Geometry check sheet. Reference: drawing and pictorial views, mm from the part's lowest x, y, z. A direction names the side the tool comes from. Give positions to 0.01 mm unless a question says otherwise; leave off trailing zeros. Write each loop counter-clockwise with the first axis right and the second up, starting at its lowest first coordinate (ties: lowest second). Pieces come first, ordered by that corner, then holes. Notation, with made-up numbers: (-9.75, 84.5) -> (39.25, 84.5) arc R12 cw to (39.25, 88.5) -> close; hole circle Ø3 at (57.25, 27.25). An arc over 180 degrees is marked (long way). Return JSON: item names as keys, results as strings.
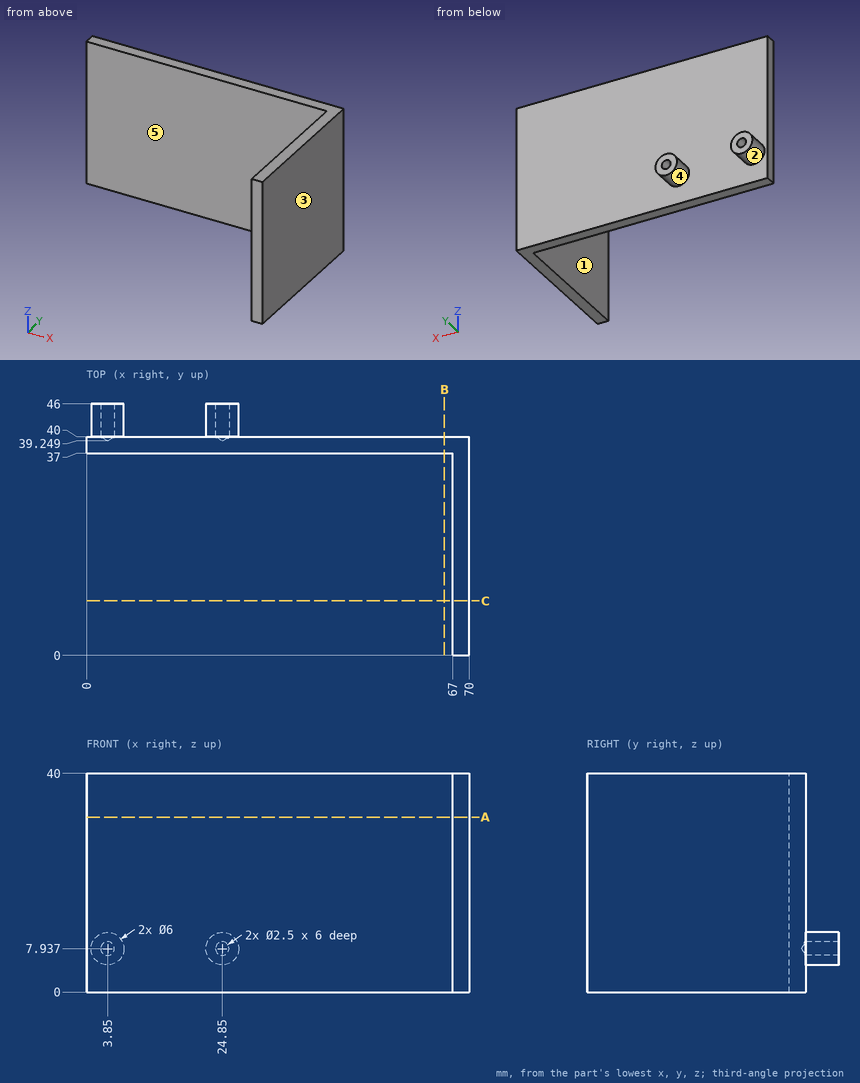
(1) Depth check by flat-ended pin: pin 1 Ø4 at (x, z) = (3.85, 7.94) entering from -Y; pin 2 Ø5 at (y, z) = (28.5, 33) entering from -X; pin 3 Ø6 at (x, z) = (46.5, 20.5) entering from +Y. Enter the tip coordinate at first touch or a pass-through.
Reply:
{"pin 1": "y = 37", "pin 2": "x = 67", "pin 3": "y = 40"}
(2) Thickness scan on L1, parallel to X at y = 28, z = 26; L2, parallel to Y at x = 17, z = 37. Record the ranges inside material, lowest first.
Reply:
{"L1": "67 to 70", "L2": "37 to 40"}
(3) Cross-section at C-C on y = 10. Enter the section's corners in (x, z).
Reply:
{"outline": "(67, 0) -> (70, 0) -> (70, 40) -> (67, 40) -> close"}
(4) Cross-section at A-A on z = 32. Enter the section's corners in (x, y), then the cut area to 3 significant figures.
Reply:
{"outline": "(0, 37) -> (67, 37) -> (67, 0) -> (70, 0) -> (70, 40) -> (0, 40) -> close", "area": "321 mm^2"}
(5) Cross-section at B-B on x = 65.5. Enter the section's corners in (y, z).
Reply:
{"outline": "(37, 0) -> (40, 0) -> (40, 40) -> (37, 40) -> close"}
(6) Set-up check for the marked faces 4 and 5: record each of +Z, -Z, +X, -X, +Y, -Y from which the full face is reachable in a straight line by a thin tool's end or side.
Reply:
{"face 4": "+Y", "face 5": "+Z, -Z, -X, -Y"}
(7) Release check for a two-part mould opening along X. For the marked faces 1, 2 and 3 record: pulls with the +X half, pulls with the -X half, needs draft (parallel to the pull), parting line crosses it, or undercut.
Reply:
{"face 1": "pulls with the -X half", "face 2": "undercut", "face 3": "pulls with the +X half"}
